```python
from build123d import *

# Parameters (mm, degrees)
SCHIZZO1_W                         = 25.92
SCHIZZO1_H                         = 31.58
ESTRUSIONE_ESTRUSIONE1_DEPTH       = 6.07
TAGLIO_ESTRUSIONE1_DEPTH           = 22.310340213
SCHIZZO3_W                         = 0.215
SCHIZZO3_H                         = 15.85
TAGLIO_ESTRUSIONE2_DEPTH           = 31.951823856
FORO_FILETTATO_M3X0_5_1_D          = 2.5
FORO_FILETTATO_M3X0_5_1_DEPTH      = 8.5
FORO_FILETTATO_M3X0_5_1_TIP        = 0.751075774
FORO_FILETTATO_M3X0_5_3_AT_2_COUNT = 2
FORO_FILETTATO_M3X0_5_3_AT_2_PITCH = 24.5


with BuildPart() as part:
    # Schizzo1 → Estrusione-Estrusione1 (new body)
    with BuildSketch(Plane.XY):
        Rectangle(SCHIZZO1_W, SCHIZZO1_H)
    extrude(amount=-ESTRUSIONE_ESTRUSIONE1_DEPTH)

    # Schizzo2 → Taglio-Estrusione1 (cut, through all)
    with BuildSketch(Plane.XY):
        Polygon((-11, 8.415), (-12.96, 9.37), (-12.96, -8.39), (-11, -7.435), align=None)
        with BuildLine():
            Line((-6.555, 5.24), (-6.555, -4.26))
            ThreePointArc((-6.555, -4.26), (-5.03, -5.785), (-3.505, -4.26))
            Line((-3.505, -4.26), (-3.505, 5.24))
            ThreePointArc((-3.505, 5.24), (-5.03, 6.765), (-6.555, 5.24))
        make_face()
        with BuildLine():
            ThreePointArc((6.555, -4.26), (5.03, -5.785), (3.505, -4.26))
            Line((3.505, -4.26), (3.505, 5.24))
            ThreePointArc((3.505, 5.24), (5.03, 6.765), (6.555, 5.24))
            Line((6.555, 5.24), (6.555, -4.26))
        make_face()
        Polygon((12.96, -8.39), (12.96, 9.37), (11, 8.415), (11, -7.435), align=None)
        with BuildLine():
            Line((-4.05, -13.34), (4.05, -13.34))
            ThreePointArc((4.05, -13.34), (5.57, -11.82), (4.05, -10.3))
            Line((4.05, -10.3), (-4.05, -10.3))
            ThreePointArc((-4.05, -10.3), (-5.57, -11.82), (-4.05, -13.34))
        make_face()
    extrude(amount=-TAGLIO_ESTRUSIONE1_DEPTH, mode=Mode.SUBTRACT)

    # Schizzo3 → Taglio-Estrusione2 (cut, through all)
    with BuildSketch(Plane.ZY.offset(12.96)):
        with Locations((-5.9625, 0.49)):
            Rectangle(SCHIZZO3_W, SCHIZZO3_H)
        with Locations((-0.1075, 0.49)):
            Rectangle(SCHIZZO3_W, SCHIZZO3_H)
    extrude(amount=-TAGLIO_ESTRUSIONE2_DEPTH, mode=Mode.SUBTRACT)

    # Foro filettato M3x0.5-1
    with Locations(Plane(origin=(0, 15.79, 0), x_dir=(1, 0, 0), z_dir=(0, 1, 0))):
        with Locations((-4, 3.035), (4, 3.035)):
            Hole(FORO_FILETTATO_M3X0_5_1_D / 2, depth=FORO_FILETTATO_M3X0_5_1_DEPTH)
            with Locations((0, 0, -(FORO_FILETTATO_M3X0_5_1_DEPTH + FORO_FILETTATO_M3X0_5_1_TIP / 2))):  # 118° drill point
                Cone(0, FORO_FILETTATO_M3X0_5_1_D / 2, FORO_FILETTATO_M3X0_5_1_TIP, mode=Mode.SUBTRACT)

    # Schizzo8 → Foro filettato M3x0.5-3 (revolve, cut)
    with BuildSketch(Plane(origin=(-12.96, 12.79, -3.035), x_dir=(0, 0, 1), z_dir=(0, 1, 0))):
        Polygon((0, 0), (0, 9.251075774), (1.25, 8.5), (1.25, 0), align=None)
    foro_filettato_m3x0_5_3 = revolve(axis=Axis((-19.31, 12.79, -3.035), (1, 0, 0)), mode=Mode.SUBTRACT)

    # Foro filettato M3x0.5-3 at 2: Foro filettato M3x0.5-3 ×2
    with Locations(*[(0, -i * FORO_FILETTATO_M3X0_5_3_AT_2_PITCH, 0) for i in range(1, FORO_FILETTATO_M3X0_5_3_AT_2_COUNT)]):
        add(foro_filettato_m3x0_5_3, mode=Mode.SUBTRACT)

    # Specchia1: Foro filettato M3x0.5-3 across plane
    add(foro_filettato_m3x0_5_3.mirror(Plane(origin=(0, 0, 0), x_dir=(0, 0, 1), z_dir=(1, 0, 0))), mode=Mode.SUBTRACT)

    # Specchia1 copy 1 sketch → Specchia1 copy 1 (revolve, cut)
    with BuildSketch(Plane(origin=(12.96, -11.71, -3.035), x_dir=(0, 0, 1), z_dir=(0, 1, 0))):
        Polygon((0, 0), (0, -9.251075774), (1.25, -8.5), (1.25, 0), align=None)
    revolve(axis=Axis((19.31, -11.71, -3.035), (1, 0, 0)), mode=Mode.SUBTRACT)


solid = part.part
```
Model file for the job. Use its own axes, mm. A direction names the side the tool comes from. Give positions to 0.01 mm unless a question says otherwise; leave off trailing zeros. Write each loop counter-clockwise with the first axis right and the second up, starting at its lowest first coordinate (ties: lowest second). Pieces come first, ordered by that corner, then holes. Notation, with made-up numbers: M 83,0 L 131,0 A24 ccw 131,21 Z; hole C 67.25,-14 d1. An arc over 180 degrees is marked long. Use a Markdown table: item, result.
1) Pin check, flat tips, straight feed: pin 1 (2 mm diameter, centred on y = -6, z = -5.5, fed in from -X); pin 2 (10 mm diameter, centred on x = -2.5, y = -10.5, fed in from +Z); pin 3 (3 mm diameter, centred on x = -10, y = 0.5, fed in from +Z) (3 decimals); pin 4 (3 mm diameter, centred on y = 3, z = -4, fed in from +X). Stop position of each tip, or through.
Responses:
| item | result |
|---|---|
| pin 1 | stops at x = -11 |
| pin 2 | stops at z = 0 |
| pin 3 | stops at z = -0.215 |
| pin 4 | stops at x = 11 |
2) Cut at A-A (z = -5.5). List the corners of the cut face in (x, y) (3 decimals).
Responses:
| item | result |
|---|---|
| outline | M -12.96,-15.79 L 12.96,-15.79 L 12.96,-8.39 L 11,-7.435 L 11,8.415 L 12.96,9.37 L 12.96,15.79 L -12.96,15.79 L -12.96,9.37 L -11,8.415 L -11,-7.435 L -12.96,-8.39 Z; hole M -6.555,-4.26 A1.525 ccw -3.505,-4.26 L -3.505,5.24 A1.525 ccw -6.555,5.24 Z; hole M -4.05,-13.34 L 4.05,-13.34 A1.52 ccw 4.05,-10.3 L -4.05,-10.3 A1.52 ccw Z; hole M 3.505,-4.26 A1.525 ccw 6.555,-4.26 L 6.555,5.24 A1.525 ccw 3.505,5.24 Z |
3) Tool access for faces 1 (the flat face through (0, 0, -5.855)), 2 (the flat face through (-11.966, 8.886, -2.993)), 3 (the cylindrical face through (-5.064, -5.785, -2.996)), 4 (the flat face through (11.994, 8.899, -2.993)): list every direction of +Z, -Z, +X, -X, +Y, -Y with a clear straight run to the whole face (end or side of a thin tool).
Responses:
| item | result |
|---|---|
| face 1 | -Z, +X, -X |
| face 2 | +Z, -Z, -X |
| face 3 | +Z, -Z |
| face 4 | +Z, -Z, +X |
4) Cut at B-B (y = 4.5). List the corners of the cut face in (x, z) (3 decimals).
Responses:
| item | result |
|---|---|
| outline | M -11,-5.855 L -6.555,-5.855 L -6.555,-0.215 L -11,-0.215 Z; M -3.505,-5.855 L 3.505,-5.855 L 3.505,-0.215 L -3.505,-0.215 Z; M 6.555,-5.855 L 11,-5.855 L 11,-0.215 L 6.555,-0.215 Z |
5) Pull direction Y, two halves, no side cores. Call faces 5 (the cylindrical face through (-2.75, 11.48, -3.09)), 6 (the flat face through (11.966, -7.906, -2.993)), 7 (the conical face through (-4, 6.7, -3.3)): +Y half, -Y half, draft (parallel to the pull), parting line (faces both ways), or undercut.
Responses:
| item | result |
|---|---|
| face 5 | draft |
| face 6 | undercut |
| face 7 | +Y half |
6) Cut at D-D (y = 12.79). List the corners of the cut face in (x, z) (3 decimals), and give its area (3 significant figures).
Responses:
| item | result |
|---|---|
| outline | M -12.96,-6.07 L 12.96,-6.07 L 12.96,-4.285 L 4.46,-4.285 L 4.417,-4.213 A1.25 cw long 4.417,-1.857 L 4.46,-1.785 L 12.96,-1.785 L 12.96,0 L -12.96,0 L -12.96,-1.785 L -4.46,-1.785 L -4.417,-1.857 A1.25 cw long -4.417,-4.213 L -4.46,-4.285 L -12.96,-4.285 Z |
| area | 108 mm2 |
7) Drill centre lines: line 1 (X direction, y = 4, z = -1) (3 decimals); line 2 (Y direction, x = -2.75, z = -6) (3 decimals); line 3 (Z direction, x = -10.75, y = 12.79) (3 decimals). Where is each one in solid material? Low to high. Write a range as from..to.
Responses:
| item | result |
|---|---|
| line 1 | x = -11..-6.555, -3.505..3.505, 6.555..11 |
| line 2 | y = -15.79..-13.34, -10.3..-7.435, 8.415..15.79 |
| line 3 | z = -6.07..-4.285, -1.785..0 |
8) Cut at C-C (x = -8). List the corners of the cut face in (y, z) (3 decimals).
Responses:
| item | result |
|---|---|
| outline | M -15.79,-6.07 L -7.435,-6.07 L -7.435,-5.855 L 8.415,-5.855 L 8.415,-6.07 L 15.79,-6.07 L 15.79,0 L 8.415,0 L 8.415,-0.215 L -7.435,-0.215 L -7.435,0 L -15.79,0 Z; hole C -11.71,-3.035 d2.5; hole C 12.79,-3.035 d2.5 |
